Model file for the job. Use its own axes, mm. A direction names the side the tool comes from. Round coordinates to 2 decimals unless told otherwise and drop trailing zeros. Order: outer loops, then holes, each group sorted by start corner. A loop starts at its lowest first (then second) coordinate and runs counter-clockwise, first axis right, second up. Notation, with made-up numbers: (-17.75, 63.25) - (-11.75, 63.25) arc R16 ccw to (-11.75, 74.25) - close; hole circle Ø2 at (-33, 11.5). An arc over 180 degrees is marked (long way). Write item = value, one per line. Start each with the question number.
from build123d import *

# Parameters (mm, degrees)
CROQUIS1_W              = 60
CROQUIS1_H              = 160.023288417
SALIENTE_EXTRUIR1_DEPTH = 7.9375
CROQUIS2_W              = 8.086078182
CROQUIS2_H              = 420
SALIENTE_EXTRUIR2_DEPTH = 110
CORTAR_EXTRUIR1_DEPTH   = 10


with BuildPart() as part:
    # Croquis1 → Saliente-Extruir1 (new body)
    # profile 1 of 2: a face of its own
    with BuildSketch(Plane(origin=(0, 0, 0), x_dir=(1, 0, 0), z_dir=(0, 1, 0))):
        Polygon((75, 210), (-75, 210), (-75, 49.976711583), (-75, -210), (75, -210), align=None)
        with BuildLine():
            ThreePointArc((-42.626797059, -194.544827159), (-50.012947046, -201.930977146), (-57.399097033, -194.544827159))
            Line((-57.399097033, -194.544827159), (-57.399097033, -162.050045053))
            ThreePointArc((-57.399097033, -162.050045053), (-50.012947046, -154.663895066), (-42.626797059, -162.050045053))
            Line((-42.626797059, -162.050045053), (-42.626797059, -194.544827159))
        make_face(mode=Mode.SUBTRACT)
        with BuildLine():
            ThreePointArc((-42.626797059, -64.544827159), (-50.012947046, -71.930977146), (-57.399097033, -64.544827159))
            Line((-57.399097033, -64.544827159), (-57.399097033, -32.050045053))
            ThreePointArc((-57.399097033, -32.050045053), (-50.012947046, -24.663895066), (-42.626797059, -32.050045053))
            Line((-42.626797059, -32.050045053), (-42.626797059, -64.544827159))
        make_face(mode=Mode.SUBTRACT)
        with BuildLine():
            ThreePointArc((57.373202941, -194.544827159), (49.987052954, -201.930977146), (42.600902967, -194.544827159))
            Line((42.600902967, -194.544827159), (42.600902967, -162.050045053))
            ThreePointArc((42.600902967, -162.050045053), (49.987052954, -154.663895066), (57.373202941, -162.050045053))
            Line((57.373202941, -162.050045053), (57.373202941, -194.544827159))
        make_face(mode=Mode.SUBTRACT)
        with BuildLine():
            ThreePointArc((57.373202941, -64.544827159), (49.987052954, -71.930977146), (42.600902967, -64.544827159))
            Line((42.600902967, -64.544827159), (42.600902967, -32.050045053))
            ThreePointArc((42.600902967, -32.050045053), (49.987052954, -24.663895066), (57.373202941, -32.050045053))
            Line((57.373202941, -32.050045053), (57.373202941, -64.544827159))
        make_face(mode=Mode.SUBTRACT)
        with BuildLine():
            ThreePointArc((-66.642728039, 194.133584854), (-61.642728039, 199.133584854), (-56.642728039, 194.133584854))
            Line((-56.642728039, 194.133584854), (-56.642728039, 74.133584854))
            ThreePointArc((-56.642728039, 74.133584854), (-61.642728039, 69.133584854), (-66.642728039, 74.133584854))
            Line((-66.642728039, 74.133584854), (-66.642728039, 194.133584854))
        make_face(mode=Mode.SUBTRACT)
    # profile 2 of 2: a face of its own
    with BuildSketch(Plane(origin=(0, 0, 0), x_dir=(1, 0, 0), z_dir=(0, 1, 0))):
        with Locations((-105, 129.988355791)):
            Rectangle(CROQUIS1_W, CROQUIS1_H)
        with BuildLine():
            ThreePointArc((-123.366972213, 194.743931483), (-118.366972213, 199.743931483), (-113.366972213, 194.743931483))
            Line((-113.366972213, 194.743931483), (-113.366972213, 74.743931483))
            ThreePointArc((-113.366972213, 74.743931483), (-118.366972213, 69.743931483), (-123.366972213, 74.743931483))
            Line((-123.366972213, 74.743931483), (-123.366972213, 194.743931483))
        make_face(mode=Mode.SUBTRACT)
    extrude(amount=SALIENTE_EXTRUIR1_DEPTH)

    # Croquis2 → Saliente-Extruir2 (add)
    with BuildSketch(Plane.XZ):
        with Locations((4.043039091, 0)):
            Rectangle(CROQUIS2_W, CROQUIS2_H)
    extrude(amount=SALIENTE_EXTRUIR2_DEPTH)

    # Croquis3 → Cortar-Extruir1 (cut)
    with BuildSketch(Plane.ZY):
        with BuildLine():
            Line((-185.90944112, -54.927638628), (-185.90944112, -94.927638628))
            ThreePointArc((-185.90944112, -94.927638628), (-192.40944112, -101.427638628), (-198.90944112, -94.927638628))
            Line((-198.90944112, -94.927638628), (-198.90944112, -54.927638628))
            ThreePointArc((-198.90944112, -54.927638628), (-192.40944112, -48.427638628), (-185.90944112, -54.927638628))
        make_face()
        with BuildLine():
            Line((-125.90944112, -54.927638628), (-125.90944112, -94.927638628))
            ThreePointArc((-125.90944112, -94.927638628), (-132.40944112, -101.427638628), (-138.90944112, -94.927638628))
            Line((-138.90944112, -94.927638628), (-138.90944112, -54.927638628))
            ThreePointArc((-138.90944112, -54.927638628), (-132.40944112, -48.427638628), (-125.90944112, -54.927638628))
        make_face()
        with BuildLine():
            Line((-65.90944112, -54.927638628), (-65.90944112, -94.927638628))
            ThreePointArc((-65.90944112, -94.927638628), (-72.40944112, -101.427638628), (-78.90944112, -94.927638628))
            Line((-78.90944112, -94.927638628), (-78.90944112, -54.927638628))
            ThreePointArc((-78.90944112, -54.927638628), (-72.40944112, -48.427638628), (-65.90944112, -54.927638628))
        make_face()
        with BuildLine():
            Line((-5.90944112, -54.927638628), (-5.90944112, -94.927638628))
            ThreePointArc((-5.90944112, -94.927638628), (-12.40944112, -101.427638628), (-18.90944112, -94.927638628))
            Line((-18.90944112, -94.927638628), (-18.90944112, -54.927638628))
            ThreePointArc((-18.90944112, -54.927638628), (-12.40944112, -48.427638628), (-5.90944112, -54.927638628))
        make_face()
        with BuildLine():
            Line((54.09055888, -54.927638628), (54.09055888, -94.927638628))
            ThreePointArc((54.09055888, -94.927638628), (47.59055888, -101.427638628), (41.09055888, -94.927638628))
            Line((41.09055888, -94.927638628), (41.09055888, -54.927638628))
            ThreePointArc((41.09055888, -54.927638628), (47.59055888, -48.427638628), (54.09055888, -54.927638628))
        make_face()
        with BuildLine():
            Line((114.09055888, -54.927638628), (114.09055888, -94.927638628))
            ThreePointArc((114.09055888, -94.927638628), (107.59055888, -101.427638628), (101.09055888, -94.927638628))
            Line((101.09055888, -94.927638628), (101.09055888, -54.927638628))
            ThreePointArc((101.09055888, -54.927638628), (107.59055888, -48.427638628), (114.09055888, -54.927638628))
        make_face()
        with BuildLine():
            Line((174.09055888, -54.927638628), (174.09055888, -94.927638628))
            ThreePointArc((174.09055888, -94.927638628), (167.59055888, -101.427638628), (161.09055888, -94.927638628))
            Line((161.09055888, -94.927638628), (161.09055888, -54.927638628))
            ThreePointArc((161.09055888, -54.927638628), (167.59055888, -48.427638628), (174.09055888, -54.927638628))
        make_face()
    extrude(amount=-CORTAR_EXTRUIR1_DEPTH, mode=Mode.SUBTRACT)


solid = part.part
Item 1: Drop flat-ended pins along their axis: pin 1 (3 mm diameter, centred on y = -9.5, z = 120.5, fed in from -X); pin 2 (2.5 mm diameter, centred on x = -104, y = 4.5, fed in from +Z); pin 3 (4 mm diameter, centred on y = 2.5, z = 127, fed in from -X). Give the stop position or say it passes through.
Item 2: Probe L1, parallel to X at y = 0.5, z = 63.5; L2, parallel to X at y = -91, z = -61.5; L3, parallel to Y at x = 9.5, z = -147.5. List the from-to ranges inside material, lowest first.
Item 3: Saw through at B-B, the plane y = -86.5. Give the number of separate pieces and of enclosed holes in the cut face, then the cut area to 3 significant figures.
Item 4: Saw through at A-A, the plane z = -168. Give the cut face in (x, y), then the cut area to 3 significant figures.
Item 5: Saw through at C-C, the plane x = -48. Give the cut face in (y, z).
Item 6: Which spindle directions (+Z, -Z, +X, -X, +Y, -Y) get a long thin tool onto all of the face, cutting with end or side? Do faces 1 (the face through (-42.627, 4, 178)), 2 (the face through (8.086, -54, -3)), 3 (the face through (4, -75, -185.909)), 4 (the face through (-75, 4, 78)). Say none if no direction does.
Item 7: Mould opens along Y. For faces 5 (the face through (-8, 7.938, -50)), 6 (the face through (-61.533, 3.913, -69.135)), 7 (the face through (4, -75, 54.091)), 8 (the face through (4, -75, 101.091)) say: +Y half, -Y half, draft (parallel to the pull), parting line (faces both ways), or undercut.
Item 8: Saw through at D-D, the plane z = 105. Give the cut face in (x, y).
Check sheet entries:
q1.pin_1 = 0
q1.pin_2 = -49.98
q1.pin_3 = -75
q2.L1 = -75 to -57.4, -42.63 to 42.6, 57.37 to 75
q2.L2 = 0 to 8.09
q2.L3 = 0 to 7.94
q3.separate_pieces = 8
q3.enclosed_holes = 0
q3.area = 2,660 mm2
q4.outline = (-135, 0) - (-123.37, 0) - (-123.37, 7.94) - (-135, 7.94) - close; (-113.37, 0) - (-66.64, 0) - (-66.64, 7.94) - (-113.37, 7.94) - close; (-56.64, 0) - (0, 0) - (0, -110) - (8.09, -110) - (8.09, 0) - (75, 0) - (75, 7.94) - (-56.64, 7.94) - close
q4.area = 2,400 mm2
q5.outline = (0, -210) - (7.94, -210) - (7.94, 24.94) - (0, 24.94) - close; (0, 71.65) - (7.94, 71.65) - (7.94, 154.94) - (0, 154.94) - close; (0, 201.65) - (7.94, 201.65) - (7.94, 210) - (0, 210) - close
q6.face_1 = +Y, -Y
q6.face_2 = +Z, -Z, +X, -Y
q6.face_3 = +X, -X
q6.face_4 = +Z, -X, +Y, -Y
q7.face_5 = +Y half
q7.face_6 = draft
q7.face_7 = undercut
q7.face_8 = undercut
q8.outline = (-75, 0) - (0, 0) - (0, -48.97) - (8.09, -48.97) - (8.09, 0) - (75, 0) - (75, 7.94) - (-75, 7.94) - close; (0, -110) - (8.09, -110) - (8.09, -100.89) - (0, -100.89) - close
